```python
from build123d import *

# Parameters (mm, degrees)
SKETCH1_W           = 300
SKETCH1_H           = 100
BOSS_EXTRUDE1_DEPTH = 20
SKETCH1_3_W         = 255
SKETCH1_3_H         = 35
BOSS_EXTRUDE2_DEPTH = 55
SKETCH1_5_W         = 60
SKETCH1_5_H         = 40
BOSS_EXTRUDE3_DEPTH = 60
CUT_EXTRUDE1_START  = 20
SKETCH1_6_W         = 120
SKETCH1_6_H         = 25
CUT_EXTRUDE1_DEPTH  = 15


with BuildPart() as part:
    # Sketch1 → Boss-Extrude1 (new body)
    with BuildSketch(Plane(origin=(0, 0, 0), x_dir=(1, 0, 0), z_dir=(0, 1, 0))):
        Rectangle(SKETCH1_W, SKETCH1_H)
    extrude(amount=BOSS_EXTRUDE1_DEPTH)

    # Sketch1<3> → Boss-Extrude2 (add)
    with BuildSketch(Plane(origin=(0, 0, 0), x_dir=(1, 0, 0), z_dir=(0, 1, 0))):
        with Locations((-22.5, -32.5)):
            Rectangle(SKETCH1_3_W, SKETCH1_3_H)
    extrude(amount=BOSS_EXTRUDE2_DEPTH)

    # Sketch1<5> → Boss-Extrude3 (add)
    with BuildSketch(Plane(origin=(0, 0, 0), x_dir=(1, 0, 0), z_dir=(0, 1, 0))):
        with Locations((120, 30)):
            Rectangle(SKETCH1_5_W, SKETCH1_5_H)
    extrude(amount=BOSS_EXTRUDE3_DEPTH)

    # Sketch1<6> → Cut-Extrude1 (cut)
    with BuildSketch(Plane(origin=(0, 0, 0), x_dir=(1, 0, 0), z_dir=(0, 1, 0)).offset(CUT_EXTRUDE1_START)):
        with Locations((-90, 37.5)):
            Rectangle(SKETCH1_6_W, SKETCH1_6_H)
    extrude(amount=-CUT_EXTRUDE1_DEPTH, mode=Mode.SUBTRACT)


solid = part.part
```
Model file for the job. Use its own axes, mm. A direction names the side the tool comes from. Round coordinates to 2 decimals unless told otherwise and drop trailing zeros. Write each loop counter-clockwise with the first axis right and the second up, starting at its lowest first coordinate (ties: lowest second). Pieces come first, ordered by that corner, then holes. Notation, with made-up numbers: (-9.75, 14.25) -> (43.25, 14.25) arc R5 cw to (43.25, 20.25) -> close; hole circle Ø3 at (52.5, 86). An arc over 180 degrees is marked (long way). Answer as CSV lines item,"result".
1. Mould opens along Z. For faces 1 (the face through (90, 40, -30)), 2 (the face through (-2, 27, 50)), 3 (the face through (120, 40, -10)) say: +Z half, -Z half, draft (parallel to the pull), parting line (faces both ways), or undercut.
Resolved:
face 1,"draft"
face 2,"+Z half"
face 3,"undercut"
2. Slice it at D-D, the plane z = 24.5. List the corners of the cut face in (x, y), plus the area to 3 significant figures.
Resolved:
outline,"(-150, 0) -> (150, 0) -> (150, 20) -> (105, 20) -> (105, 55) -> (-150, 55) -> close"
area,"14,900 mm²"
3. Slice it at B-B, the plane x = -128.5. List the corners of the cut face in (y, z), plus the area to 3 significant figures.
Resolved:
outline,"(0, -50) -> (5, -50) -> (5, -25) -> (20, -25) -> (20, 15) -> (55, 15) -> (55, 50) -> (0, 50) -> close"
area,"2,850 mm²"
4. Slice it at C-C, the plane z = -39. List the corners of the cut face in (x, y), plus the area to 3 significant figures.
Resolved:
outline,"(-150, 0) -> (150, 0) -> (150, 60) -> (90, 60) -> (90, 20) -> (-30, 20) -> (-30, 5) -> (-150, 5) -> close"
area,"6,600 mm²"
5. Slice it at A-A, the plane y = 25.5. List the corners of the cut face in (x, z), plus the area to 3 significant figures.
Resolved:
outline,"(-150, 15) -> (105, 15) -> (105, 50) -> (-150, 50) -> close; (90, -50) -> (150, -50) -> (150, -10) -> (90, -10) -> close"
area,"11,300 mm²"
6. Drill centre lines: line 1 (Z direction, x = 103, y = 40); line 2 (Y direction, x = -129, z = -29.5); line 3 (X direction, y = 35, z = 29). Where is each one in solid material? Low to high.
Resolved:
line 1,"-50 to -10, 15 to 50"
line 2,"0 to 5"
line 3,"-150 to 105"
7. Pin check, flat tips, straight feed: pin 1 Ø12 at (x, y) = (-60, 13.5) entering from -Z; pin 2 Ø10.5 at (x, y) = (-83.5, 31) entering from -Z; pin 3 Ø17.5 at (x, z) = (23, 35.5) entering from +Y. Stop position of each tip, or through.
Resolved:
pin 1,"z = -25"
pin 2,"z = 15"
pin 3,"y = 55"
8. Tool access for faces 4 (the face through (-150, 21, 23)), 5 (the face through (-91, 5, -38)), 6 (the face through (105, 37, 33)): list every direction of +Z, -Z, +X, -X, +Y, -Y with a clear straight run to the whole face (end or side of a thin tool).
Resolved:
face 4,"+Z, -Z, -X, +Y, -Y"
face 5,"-Z, -X, +Y"
face 6,"+Z, +X, +Y"
